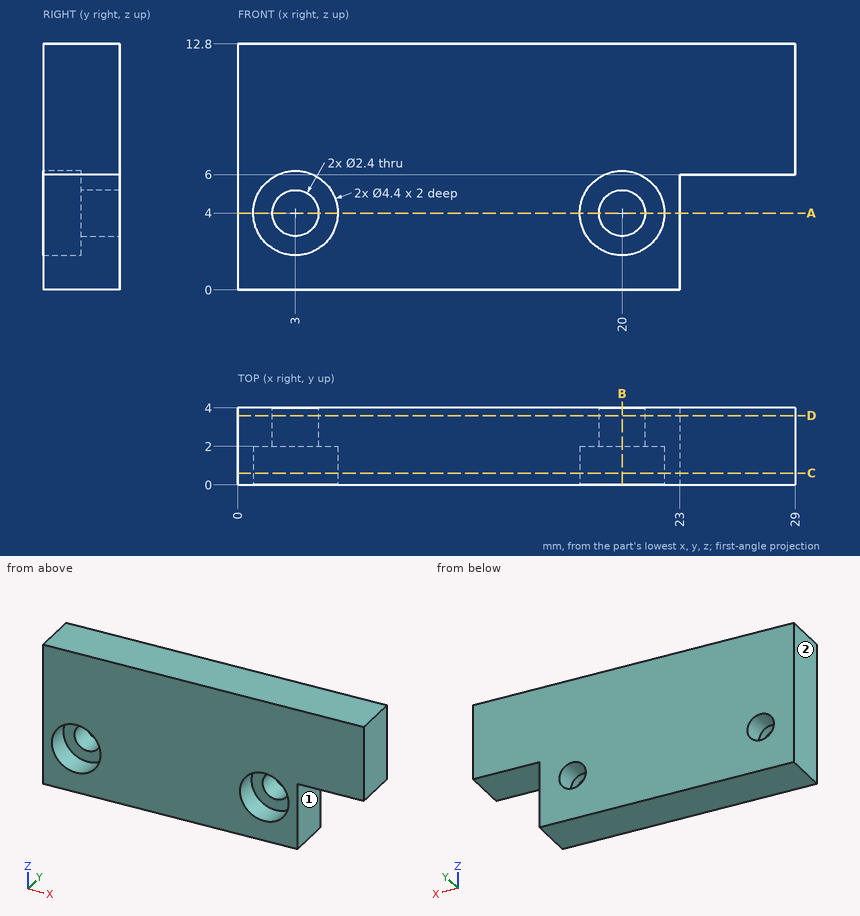
Geometry: see drawing. Coordinates: mm, zero at the bounding-box minimum. A direction names the side the tool comes from. Round coordinates to 2 decimals unless told otherwise and drop trailing zeros. Order: outer loops, then holes, each group sorted by start corner. A loop starts at its lowest first (then second) coordinate and runs counter-clockwise, first axis right, second up. Notation, with made-up numbers: (13.25, 37) -> (39.25, 37) arc R35 ccw to (39.25, 71) -> close; hole circle Ø8 at (68.5, 28.25). An arc over 180 degrees is marked (long way). Write each question's results on one line, items separated by ' | '.
Q1. Section query D-D (y = 3.6). Output: boundary loops of the cut face in (x, z), and give its area (3 significant figures).
Response values:
outline: (0, 0) -> (23, 0) -> (23, 6) -> (29, 6) -> (29, 12.8) -> (0, 12.8) -> close; hole circle Ø2.4 at (3, 4); hole circle Ø2.4 at (20, 4) | area: 326 mm²
Q2. Access query for the marked faces 1 and 2. Directions: +Z, -Z, +X, -X, +Y, -Y. A direction counts if a zero-diameter tool reaches every point of the face in a straight line with its end or side. Return the directions, or none.
Response values:
face 1: -Z, +X, +Y, -Y | face 2: +Z, -Z, -X, +Y, -Y
Q3. Ray query, line 1 along X through (y, z) = (0.4, 4); line 2 along X through (y, z) = (3.4, 4); line 3 along Z through (x, y) = (3, 0.25). Return the intervals inside material, ascending.
Response values:
line 1: 0 to 0.8, 5.2 to 17.8, 22.2 to 23 | line 2: 0 to 1.8, 4.2 to 18.8, 21.2 to 23 | line 3: 0 to 1.8, 6.2 to 12.8
Q4. Section query A-A (z = 4). Output: boundary loops of the cut face in (x, y), and give its area (3 significant figures).
Response values:
outline: (0, 0) -> (0.8, 0) -> (0.8, 2) -> (1.8, 2) -> (1.8, 4) -> (0, 4) -> close; (4.2, 2) -> (5.2, 2) -> (5.2, 0) -> (17.8, 0) -> (17.8, 2) -> (18.8, 2) -> (18.8, 4) -> (4.2, 4) -> close; (21.2, 2) -> (22.2, 2) -> (22.2, 0) -> (23, 0) -> (23, 4) -> (21.2, 4) -> close | area: 64.8 mm²
Q5. Pin query (flat end, axial travel): pin 1 Ø4 at (x, z) = (20, 4) entering from -Y; pin 2 Ø1.9 at (x, z) = (3, 4) entering from -Y; pin 3 Ø1.2 at (x, y) = (24.5, 1.5) entering from -Z. Return the tip coordinate at first contact, or that it passes through.
Response values:
pin 1: y = 2 | pin 2: through | pin 3: z = 6
Q6. Section query B-B (x = 20). Output: boundary loops of the cut face in (y, z).
Response values:
outline: (0, 0) -> (4, 0) -> (4, 2.8) -> (2, 2.8) -> (2, 1.8) -> (0, 1.8) -> close; (0, 6.2) -> (2, 6.2) -> (2, 5.2) -> (4, 5.2) -> (4, 12.8) -> (0, 12.8) -> close
Q7. Section query C-C (y = 0.6). Output: boundary loops of the cut face in (x, z).
Response values:
outline: (0, 0) -> (23, 0) -> (23, 6) -> (29, 6) -> (29, 12.8) -> (0, 12.8) -> close; hole circle Ø4.4 at (3, 4); hole circle Ø4.4 at (20, 4)
